Model file for the job. Use its own axes, mm. Face numbers are marked on the shaded views. Give positions to 0.01 mm unless a question says otherwise; leave off trailing zeros. Loops run counter-clockwise (first coordinate to the right, second up) from the corner with the lowest first, then second, coordinate; pieces in that order, holes last. Notation, with made-up numbers: (52.5, 74) - (99.5, 74) arc R11 ccw to (99.5, 90) - close; hole circle Ø7 at (-9, 29.5). An arc over 180 degrees is marked (long way). Use a Markdown table: item, result.
from build123d import *

# Parameters (mm, degrees)
SALIENTE_EXTRUIR1_DEPTH = 1.5
CROQUIS2_R              = 3.5
CROQUIS2_R_2            = 2.5
SALIENTE_EXTRUIR2_DEPTH = 2.3
CROQUIS4_R              = 0.5
CORTAR_EXTRUIR1_DEPTH   = 29.964460982
CORTAR_EXTRUIR2_REACH   = 30.964
CROQUIS5_R              = 0.5


with BuildPart() as part:
    # Croquis1 → Saliente-Extruir1 (new body)
    with BuildSketch(Plane.XY):
        with BuildLine():
            Line((0, 3.5), (25, 3.5))
            ThreePointArc((25, 3.5), (28.5, 0), (25, -3.5))
            Line((25, -3.5), (0, -3.5))
            ThreePointArc((0, -3.5), (-3.5, 0), (0, 3.5))
        make_face()
    extrude(amount=SALIENTE_EXTRUIR1_DEPTH)

    # Croquis2 → Saliente-Extruir2 (add)
    with BuildSketch(Plane.XY.offset(1.5)):
        with Locations(Location((12.5, 0, 0), (0, 0, 270))):
            Circle(CROQUIS2_R)
        with Locations((12.5, 0)):
            Circle(CROQUIS2_R_2, mode=Mode.SUBTRACT)
    extrude(amount=SALIENTE_EXTRUIR2_DEPTH)

    # Croquis4 → Cortar-Extruir1 (cut, through all)
    with BuildSketch(Plane(origin=(0, 0, 0), x_dir=(-1, 0, 0), z_dir=(0, 0, -1))):
        Circle(CROQUIS4_R)
        with Locations(Location((-25, 0, 0), (0, 0, 180))):
            Circle(CROQUIS4_R)
    extrude(amount=-CORTAR_EXTRUIR1_DEPTH, mode=Mode.SUBTRACT)

    # Croquis5 → Cortar-Extruir2 (cut, up to next)
    with BuildSketch(Plane(origin=(0, 0, 0), x_dir=(-1, 0, 0), z_dir=(0, 0, -1)), mode=Mode.PRIVATE) as cortar_extruir2_sk1:
        with Locations((-8, 0)):
            Circle(CROQUIS5_R)
    cortar_extruir2_tool1 = extrude(cortar_extruir2_sk1.sketch, amount=-CORTAR_EXTRUIR2_REACH, mode=Mode.PRIVATE) & part.part
    # Croquis5 → Cortar-Extruir2 (cut, up to next)
    with BuildSketch(Plane(origin=(0, 0, 0), x_dir=(-1, 0, 0), z_dir=(0, 0, -1)), mode=Mode.PRIVATE) as cortar_extruir2_sk2:
        with Locations((-6, 0)):
            Circle(CROQUIS5_R)
    cortar_extruir2_tool2 = extrude(cortar_extruir2_sk2.sketch, amount=-CORTAR_EXTRUIR2_REACH, mode=Mode.PRIVATE) & part.part
    # Croquis5 → Cortar-Extruir2 (cut, up to next)
    with BuildSketch(Plane(origin=(0, 0, 0), x_dir=(-1, 0, 0), z_dir=(0, 0, -1)), mode=Mode.PRIVATE) as cortar_extruir2_sk3:
        with Locations((-4, 0)):
            Circle(CROQUIS5_R)
    cortar_extruir2_tool3 = extrude(cortar_extruir2_sk3.sketch, amount=-CORTAR_EXTRUIR2_REACH, mode=Mode.PRIVATE) & part.part
    # Croquis5 → Cortar-Extruir2 (cut, up to next)
    with BuildSketch(Plane(origin=(0, 0, 0), x_dir=(-1, 0, 0), z_dir=(0, 0, -1)), mode=Mode.PRIVATE) as cortar_extruir2_sk4:
        with Locations((-2, 0)):
            Circle(CROQUIS5_R)
    cortar_extruir2_tool4 = extrude(cortar_extruir2_sk4.sketch, amount=-CORTAR_EXTRUIR2_REACH, mode=Mode.PRIVATE) & part.part
    # Croquis5 → Cortar-Extruir2 (cut, up to next)
    with BuildSketch(Plane(origin=(0, 0, 0), x_dir=(-1, 0, 0), z_dir=(0, 0, -1)), mode=Mode.PRIVATE) as cortar_extruir2_sk5:
        with Locations(Location((-23, 0, 0), (0, 0, 180))):
            Circle(CROQUIS5_R)
    cortar_extruir2_tool5 = extrude(cortar_extruir2_sk5.sketch, amount=-CORTAR_EXTRUIR2_REACH, mode=Mode.PRIVATE) & part.part
    # Croquis5 → Cortar-Extruir2 (cut, up to next)
    with BuildSketch(Plane(origin=(0, 0, 0), x_dir=(-1, 0, 0), z_dir=(0, 0, -1)), mode=Mode.PRIVATE) as cortar_extruir2_sk6:
        with Locations(Location((-21, 0, 0), (0, 0, 180))):
            Circle(CROQUIS5_R)
    cortar_extruir2_tool6 = extrude(cortar_extruir2_sk6.sketch, amount=-CORTAR_EXTRUIR2_REACH, mode=Mode.PRIVATE) & part.part
    # Croquis5 → Cortar-Extruir2 (cut, up to next)
    with BuildSketch(Plane(origin=(0, 0, 0), x_dir=(-1, 0, 0), z_dir=(0, 0, -1)), mode=Mode.PRIVATE) as cortar_extruir2_sk7:
        with Locations(Location((-19, 0, 0), (0, 0, 180))):
            Circle(CROQUIS5_R)
    cortar_extruir2_tool7 = extrude(cortar_extruir2_sk7.sketch, amount=-CORTAR_EXTRUIR2_REACH, mode=Mode.PRIVATE) & part.part
    # Croquis5 → Cortar-Extruir2 (cut, up to next)
    with BuildSketch(Plane(origin=(0, 0, 0), x_dir=(-1, 0, 0), z_dir=(0, 0, -1)), mode=Mode.PRIVATE) as cortar_extruir2_sk8:
        with Locations(Location((-17, 0, 0), (0, 0, 180))):
            Circle(CROQUIS5_R)
    cortar_extruir2_tool8 = extrude(cortar_extruir2_sk8.sketch, amount=-CORTAR_EXTRUIR2_REACH, mode=Mode.PRIVATE) & part.part
    add(cortar_extruir2_tool1.solids().sort_by_distance((8, 0, 0))[0], mode=Mode.SUBTRACT)
    add(cortar_extruir2_tool2.solids().sort_by_distance((6, 0, 0))[0], mode=Mode.SUBTRACT)
    add(cortar_extruir2_tool3.solids().sort_by_distance((4, 0, 0))[0], mode=Mode.SUBTRACT)
    add(cortar_extruir2_tool4.solids().sort_by_distance((2, 0, 0))[0], mode=Mode.SUBTRACT)
    add(cortar_extruir2_tool5.solids().sort_by_distance((23, 0, 0))[0], mode=Mode.SUBTRACT)
    add(cortar_extruir2_tool6.solids().sort_by_distance((21, 0, 0))[0], mode=Mode.SUBTRACT)
    add(cortar_extruir2_tool7.solids().sort_by_distance((19, 0, 0))[0], mode=Mode.SUBTRACT)
    add(cortar_extruir2_tool8.solids().sort_by_distance((17, 0, 0))[0], mode=Mode.SUBTRACT)


solid = part.part
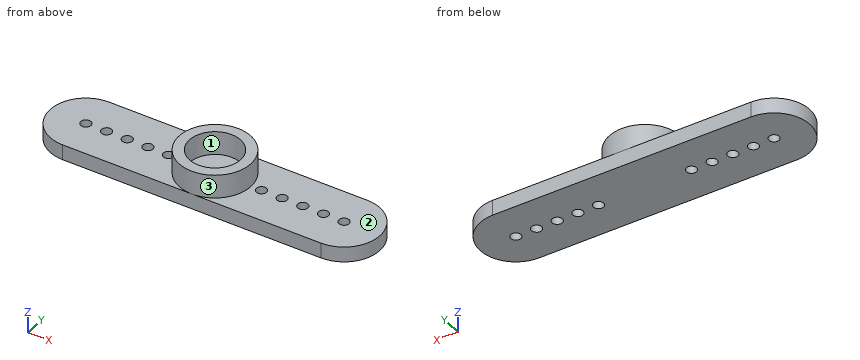
(1) Slice it at B-B, the plane y = 0. Count the separate pieces of the cut face and the enclosed holes in it, plus the area to 3 significant figures.
Computed:
| item | result |
|---|---|
| separate pieces | 11 |
| enclosed holes | 0 |
| area | 37.6 mm² |
(2) Drill centre lines: probe 1 along Y at (x, z) = (19, 0.95); probe 2 along Z at (x, y) = (5, 2.5); probe 3 along X at (y, z) = (1, 2.75). Where is each one in solid material? Low to high. Write a range as [from, to].
Computed:
| item | result |
|---|---|
| probe 1 | [-3.5, -0.5], [0.5, 3.5] |
| probe 2 | [0, 1.5] |
| probe 3 | [9.15, 10.21], [14.79, 15.85] |
(3) Slice it at D-D, the plane y = 1.5. Write the cut outline in (x, z).
Computed:
| item | result |
|---|---|
| outline | (-3.16, 0) - (28.16, 0) - (28.16, 1.5) - (15.66, 1.5) - (15.66, 3.8) - (14.5, 3.8) - (14.5, 1.5) - (10.5, 1.5) - (10.5, 3.8) - (9.34, 3.8) - (9.34, 1.5) - (-3.16, 1.5) - close |
(4) Mould opens along Y. For the marked faces 1, 2 and 3 say: pulls with the +Y half, pulls with the -Y half, needs draft (parallel to the pull), parting line crosses it, or undercut.
Computed:
| item | result |
|---|---|
| face 1 | undercut |
| face 2 | needs draft |
| face 3 | parting line crosses it |
(5) Slice it at C-C, the plane z = 3.5. Write the cut outline in (x, y).
Computed:
| item | result |
|---|---|
| outline | circle Ø7 at (12.5, 0); hole circle Ø5 at (12.5, 0) |
(6) Slice it at A-A, the plane x = 4. Write the cut outline in (y, z).
Computed:
| item | result |
|---|---|
| outline | (-3.5, 0) - (-0.5, 0) - (-0.5, 1.5) - (-3.5, 1.5) - close; (0.5, 0) - (3.5, 0) - (3.5, 1.5) - (0.5, 1.5) - close |
(7) Pin check, flat tips, straight feed: P1, Ø2, axis at y = 1, z = 3, coming from the +X side; P2, Ø3.5, axis at x = 19.5, y = 0, coming from the +Z side. Stop position of each tip, or through.
Computed:
| item | result |
|---|---|
| P1 | x = 16 |
| P2 | z = 1.5 |
